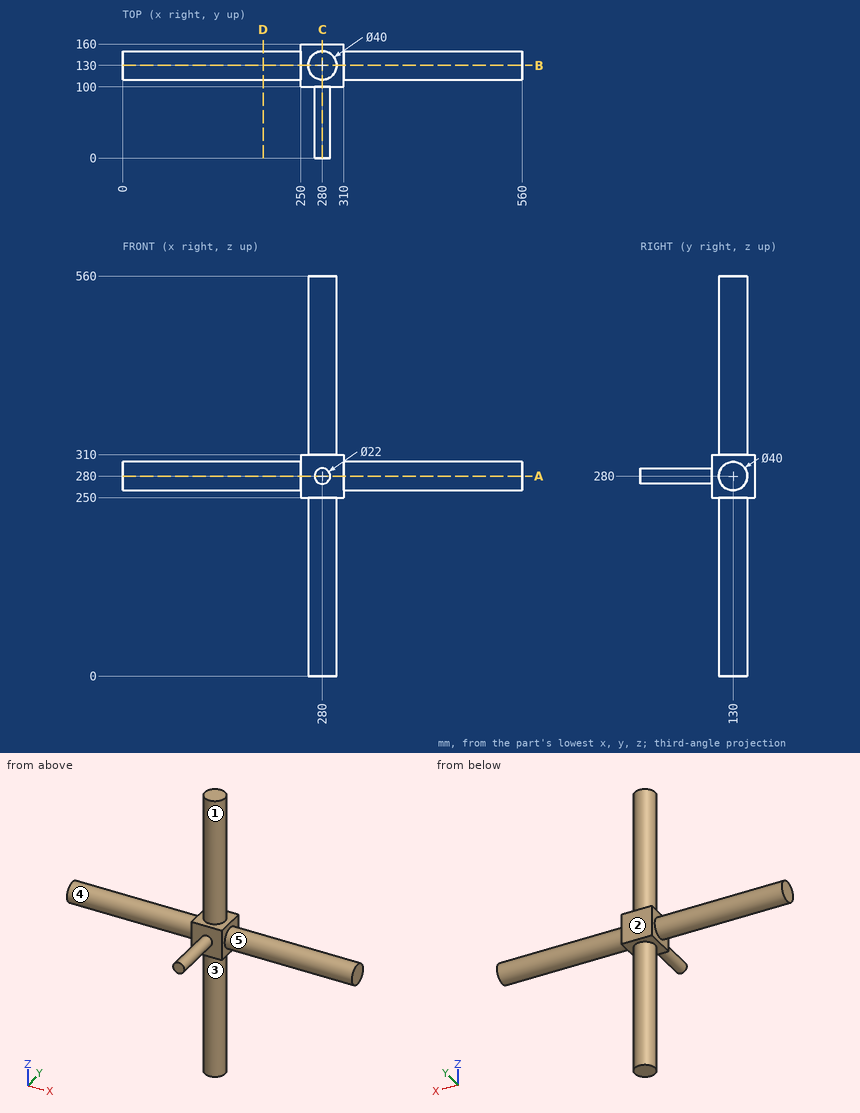
Geometry check sheet. Reference: drawing and pictorial views, mm from the part's lowest x, y, z. A direction names the side the tool comes from. Give positions to 0.01 mm unless a question says otherwise; leave off trailing zeros. Order: outer loops, then holes, each group sorted by start corner. A loop starts at its lowest first (then second) coordinate and runs counter-clockwise, first axis right, second up. Notation, with made-up numbers: (41.5, -19) - (78.5, -19) arc R24 ccw to (78.5, 6) - close; hole circle Ø1 at (-29, 40.25). An arc over 180 degrees is marked (long way). Use one line per item in the form item = value.
1) Sectioned sample at A-A (z = 280). Record the boundary of the cut face in (x, y), and give its area (3 significant figures).
Working result:
outline = (0, 110) - (250, 110) - (250, 100) - (269, 100) - (269, 0) - (291, 0) - (291, 100) - (310, 100) - (310, 110) - (560, 110) - (560, 150) - (310, 150) - (310, 160) - (250, 160) - (250, 150) - (0, 150) - close
area = 25,800 mm^2
2) Sectioned sample at C-C (x = 280). Record the boundary of the cut face in (y, z).
Working result:
outline = (0, 269) - (100, 269) - (100, 250) - (110, 250) - (110, 0) - (150, 0) - (150, 250) - (160, 250) - (160, 310) - (150, 310) - (150, 560) - (110, 560) - (110, 310) - (100, 310) - (100, 291) - (0, 291) - close
3) Depth check by flat-ended pin: pin 1 Ø1.5 at (x, y) = (355, 116) entering from -Z. Enter the tip coordinate at first touch or a pass-through.
Working result:
pin_1 = 265.02
4) Sectioned sample at B-B (y = 130). Record the boundary of the cut face in (x, z).
Working result:
outline = (0, 260) - (250, 260) - (250, 250) - (260, 250) - (260, 0) - (300, 0) - (300, 250) - (310, 250) - (310, 260) - (560, 260) - (560, 300) - (310, 300) - (310, 310) - (300, 310) - (300, 560) - (260, 560) - (260, 310) - (250, 310) - (250, 300) - (0, 300) - close
5) Material ranges on probe 1 along X at (y, z) = (123, 254.5); probe 2 along Z at (x, y) = (396.5, 134); probe 3 along X at (y, z) = (112, 495), recorded low to high. Write a range as from..to.
Working result:
probe_1 = 250..310
probe_2 = 260.4..299.6
probe_3 = 271.28..288.72
6) Sectioned sample at D-D (x = 197). Record the boundary of the cut face in (y, z).
Working result:
outline = circle Ø40 at (130, 280)
7) Access from +Z, -Z, +X, -X, +Y, -Y to the whole of each face (thin tool, end or side, straight path). Record for the marked faces 1, 2, 3, 4 and 5.
Working result:
face_1 = +Z
face_2 = +Z, -Z, +X, -X, +Y
face_3 = -Z
face_4 = -X
face_5 = +X
